Can you work these out from the model? Positions are in its coordinate system, mm. A direction names the side the tool comes from. Coordinates: 2 decimals unless noted, no trailing zeros. Write each loop counter-clockwise with the first axis right and the second up, starting at its lowest first coordinate (ties: lowest second). Pieces come first, ordered by that corner, then holes.
```python
from build123d import *

# Parameters (mm, degrees)
F0_W     = 228.6
F0_H     = 38.1
F0_R     = 12.7
F1_DEPTH = 19.05
F2_R     = 15.875
F2_R_2   = 12.7
F3_DEPTH = 12.7


with BuildPart() as f1:
    # F0 (on Top) → F1 (new body)
    with BuildSketch(Plane.XY):
        Rectangle(F0_W, F0_H)
        with Locations((-88.9, 0)):
            Circle(F0_R, mode=Mode.SUBTRACT)
        with Locations((88.9, 0)):
            Circle(F0_R, mode=Mode.SUBTRACT)
    extrude(amount=F1_DEPTH)

    # F2 (on face) → F3 (join)
    with BuildSketch(Plane.XY.offset(19.05)):
        Circle(F2_R)
        Circle(F2_R_2, mode=Mode.SUBTRACT)
    extrude(amount=F3_DEPTH)


solid = f1.part
```
1. If we section it at A-A, the plane y = 0: List the corners of the cut face in (x, z) for me (3 decimals), plus the area to 3 significant figures.
2. If I drill on L1, parallel to Y at x = 88.9, z = 14; L2, parallel to Y at x = 0, z = 26 (3 decimals); L3, parallel to Z at x = 44, y = 4.5, over which ranges is the centre line in solid material (lowest first)?
3. If we section it at D-D, the plane z = 8: List the corners of the cut face in (x, y) for me.
4. If we section it at B-B, the plane x = -88.9: List the corners of the cut face in (y, z) for me, plus the area to 3 significant figures.
5. I'm going to push flat-ended pins straight in: P1, Ø15, axis at x = -88.9, y = 0, coming from the -Z side; P2, Ø7.5, axis at x = -1.5, y = -5, coming from the +Z side. Where does each tip first touch, or does it pass through?
6. We'd pull the mould along X, two halves only. Please class faces 3 (the face through (-114.3, 0, 9)), 4 (the face through (-2, -19.05, 9)), 5 (the face through (101.014, 3.815, 9.392)): released by +X, released by -X, zero draft, split by the parting line, or undercut.
7. Which directions (+Z, -Z, +X, -X, +Y, -Y) give clear straight access to the entire face, cutting with the end or side of a thin tool? Please do faces 1 (the face through (-2, 0, 0)), 2 (the face through (0, 0, 19.05)).
8. If we section it at C-C, the plane z = 25.5: List the corners of the cut face in (x, y) for me (3 decimals).
Answers:
1. outline: (-114.3, 0) - (-101.6, 0) - (-101.6, 19.05) - (-114.3, 19.05) - close; (-76.2, 0) - (76.2, 0) - (76.2, 19.05) - (15.875, 19.05) - (15.875, 31.75) - (12.7, 31.75) - (12.7, 19.05) - (-12.7, 19.05) - (-12.7, 31.75) - (-15.875, 31.75) - (-15.875, 19.05) - (-76.2, 19.05) - close; (101.6, 0) - (114.3, 0) - (114.3, 19.05) - (101.6, 19.05) - close
1. area: 3,470 mm2
2. L1: y = -19.05 to -12.7, 12.7 to 19.05
2. L2: y = -15.875 to -12.7, 12.7 to 15.875
2. L3: z = 0 to 19.05
3. outline: (-114.3, -19.05) - (114.3, -19.05) - (114.3, 19.05) - (-114.3, 19.05) - close; hole circle Ø25.4 at (-88.9, 0); hole circle Ø25.4 at (88.9, 0)
4. outline: (-19.05, 0) - (-12.7, 0) - (-12.7, 19.05) - (-19.05, 19.05) - close; (12.7, 0) - (19.05, 0) - (19.05, 19.05) - (12.7, 19.05) - close
4. area: 242 mm2
5. P1: passes through
5. P2: stops at z = 19.05
6. face 3: released by -X
6. face 4: zero draft
6. face 5: undercut
7. face 1: -Z, +X, -X, +Y, -Y
7. face 2: +Z
8. outline: circle Ø31.75 at (0, 0); hole circle Ø25.4 at (0, 0)
